Model file for the job. Use its own axes, mm. Face numbers are marked on the shaded views. A direction names the side the tool comes from. Round coordinates to 2 decimals unless told otherwise and drop trailing zeros. Order: outer loops, then holes, each group sorted by start corner. A loop starts at its lowest first (then second) coordinate and runs counter-clockwise, first axis right, second up. Notation, with made-up numbers: (51, 53) - (62, 53) arc R27 ccw to (62, 90) - close; hole circle Ø8 at (55.5, -22). An arc over 180 degrees is marked (long way). Answer as CSV lines item,"result". Start each with the question number.
1. Band-saw the part on B-B on x = -25.5. List the corners of the cut face in (y, z).
2. Band-saw the part on D-D on x = -37. List the corners of the cut face in (y, z).
3. Wall check: line 1 along X through (y, z) = (21.5, 4.7); line 2 along Y through (x, z) = (-25, 3.85); line 3 along Y through (x, z) = (-2.5, 2.75). Give the ranges that are in metal, low to high. Write a range as [from, to].
4. Band-saw the part on A-A on y = 30.5. List the corners of the cut face in (x, z).
5. 3-axis set-ups, long thin cutter, end or side, ignore diameter. For the marked faces 4 and 5: which of +Z, -Z, +X, -X, +Y, -Y reach the whole face in a straight line?
6. Band-saw the part on C-C on y = 11. List the corners of the cut face in (x, z).
7. Pull direction Y, two halves, no side cores. Call the marked faces 1, 2 and 3: released by +Y, released by -Y, zero draft, split by the parting line, or undercut.
8. Pin check, flat tip, straight feed: pin 1 Ø5 at (x, y) = (-27.5, 19) entering from +Z. Stop position of the tip, or through.
```python
from build123d import *

# Parameters (mm, degrees)
F0_W          = 40
F0_H          = 35
F1_DEPTH      = 6
F2_W          = 16
F2_H          = 24
F3_DEPTH      = 5
F4_W          = 13
F4_H          = 3
F5_DEPTH      = 1
F5_DEPTH_BACK = 2
F6_R          = 0.5
F7_DEPTH      = 0.5
F8_W          = 13
F8_H          = 3
F9_DEPTH      = 1
F9_DEPTH_BACK = 1
F10_R         = 0.5
F10_R_2       = 0.4192188994
F11_DEPTH     = 0.5


with BuildPart() as f1:
    # F0 (on Top) → F1 (new body)
    with BuildSketch(Plane.XY):
        with Locations((-20, 17.5)):
            Rectangle(F0_W, F0_H)
    extrude(amount=F1_DEPTH)

    # F2 (on face) → F3 (cut)
    with BuildSketch(Plane.XY.offset(6)):
        with Locations((-30, 18)):
            Rectangle(F2_W, F2_H)
        with Locations((-10, 18)):
            Rectangle(F2_W, F2_H)
    extrude(amount=-F3_DEPTH, mode=Mode.SUBTRACT)

    # F4 (on face) → F5 (cut, two sides)
    with BuildSketch(Plane.XZ.offset(-30)) as f5_sk:
        with Locations((-30, 3.5)):
            Rectangle(F4_W, F4_H)
        with Locations((-10, 3.5)):
            Rectangle(F4_W, F4_H)
    extrude(amount=-F5_DEPTH, mode=Mode.SUBTRACT)
    extrude(f5_sk.sketch, amount=F5_DEPTH_BACK, mode=Mode.SUBTRACT)

    # F6 (on face) → F7 (cut)
    with BuildSketch(Plane.XZ.offset(-31)):
        with Locations((-35, 3.5)):
            Circle(F6_R)
        with Locations((-5, 3.5)):
            Circle(F6_R)
    extrude(amount=-F7_DEPTH, mode=Mode.SUBTRACT)

    # F8 (on face) → F9 (cut, two sides)
    with BuildSketch(Plane(origin=(0, 6, 0), x_dir=(-1, 0, 0), z_dir=(0, 1, 0))) as f9_sk:
        with Locations((10, 3.5)):
            Rectangle(F8_W, F8_H)
        with Locations((30, 3.5)):
            Rectangle(F8_W, F8_H)
    extrude(amount=-F9_DEPTH, mode=Mode.SUBTRACT)
    extrude(f9_sk.sketch, amount=F9_DEPTH_BACK, mode=Mode.SUBTRACT)

    # F10 (on face) → F11 (cut)
    with BuildSketch(Plane(origin=(0, 5, 0), x_dir=(-1, 0, 0), z_dir=(0, 1, 0))):
        with Locations((5.5, 3.5)):
            Circle(F10_R)
        with Locations((34.5807811006, 3.4192188994)):
            Circle(F10_R_2)
    extrude(amount=-F11_DEPTH, mode=Mode.SUBTRACT)


solid = f1.part
```
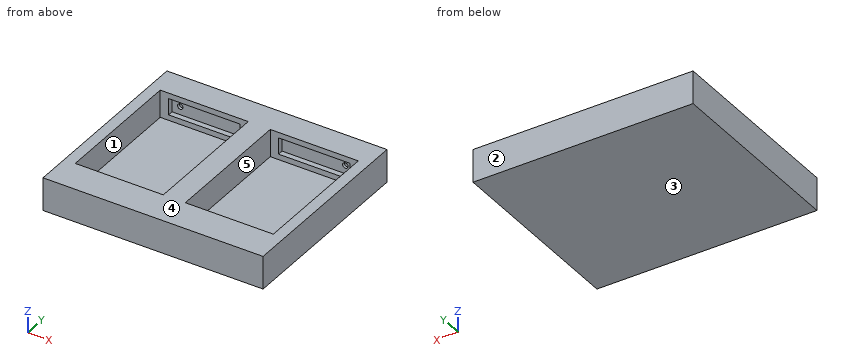
Reply:
1,outline,"(0, 0) - (35, 0) - (35, 6) - (30, 6) - (30, 5) - (31, 5) - (31, 2) - (30, 2) - (30, 1) - (6, 1) - (6, 2) - (5, 2) - (5, 5) - (6, 5) - (6, 6) - (0, 6) - close"
2,outline,"(0, 0) - (35, 0) - (35, 6) - (30, 6) - (30, 1) - (6, 1) - (6, 6) - (0, 6) - close"
3,line 1,"x = [-40, -38], [-22, -18], [-2, 0]"
3,line 2,"y = [0, 5], [31, 35]"
3,line 3,"y = [0, 6], [30, 35]"
4,outline,"(-40, 0) - (0, 0) - (0, 6) - (-40, 6) - close; hole (-36.5, 2) - (-23.5, 2) - (-23.5, 5) - (-36.5, 5) - close; hole (-16.5, 2) - (-3.5, 2) - (-3.5, 5) - (-16.5, 5) - close"
5,face 4,"+Z, +X, -X, +Y, -Y"
5,face 5,"+Z"
6,outline,"(-40, 0) - (0, 0) - (0, 6) - (-2, 6) - (-2, 1) - (-18, 1) - (-18, 6) - (-22, 6) - (-22, 1) - (-38, 1) - (-38, 6) - (-40, 6) - close"
7,face 1,"undercut"
7,face 2,"released by +Y"
7,face 3,"zero draft"
8,pin 1,"stops at z = 1"
